Input: part model. Units: mm. Frame: model coordinates. A direction names the side the tool comes from. Coordinates: 2 decimals unless noted, no trailing zeros. Loops run counter-clockwise (first coordinate to the right, second up) from the corner with the lowest first, then second, coordinate; pieces in that order, holes last. Notation, with made-up numbers: (76.25, -5) - (125.25, -5) arc R13 ccw to (125.25, 4) - close; hole circle Ø5 at (88, 70.25). An arc over 180 degrees is marked (long way). Use one line per item in the form item = value.
from build123d import *

# Parameters (mm, degrees)
SCHIZZO1_W                    = 200
SCHIZZO1_H                    = 20
ESTRUSIONE_ESTRUSIONE1_DEPTH  = 25
SCHIZZO2_R                    = 2.25
TAGLIO_ESTRUSIONE1_DEPTH      = 141.400046302
SCHIZZO4_W                    = 2.020725942
SCHIZZO4_H                    = 10
SCHIZZO4_W_2                  = 2.598076211
SCHIZZO4_W_3                  = 3.175426481
TAGLIO_ESTRUSIONE2_DEPTH      = 1
SCHIZZO7_W                    = 15
SCHIZZO7_H                    = 5.5
TAGLIO_ESTRUSIONE3_DEPTH      = 141.400046302
SMUSSO1_SIZE                  = 1.5
SMUSSO1_SIZE2                 = 6
SCHIZZO8_W                    = 25
SCHIZZO8_H                    = 2.5
TAGLIO_ESTRUSIONE4_DEPTH      = 13
SCHIZZO9_W                    = 40
SCHIZZO9_H                    = 2.5
TAGLIO_ESTRUSIONE5_DEPTH      = 141.400046302
SCHIZZO10_W                   = 7
SCHIZZO10_H                   = 3
ESTRUSIONE_ESTRUSIONE5_DEPTH  = 4
SMUSSO2_SIZE                  = 4
SCHIZZO11_W                   = 2.5
SCHIZZO11_H                   = 8
TAGLIO_ESTRUSIONE6_DEPTH      = 141.400046302
SCHIZZO12_W                   = 6.5
SCHIZZO12_H                   = 6.5
TAGLIO_ESTRUSIONE7_DEPTH      = 4
SCHIZZO13_W                   = 9
SCHIZZO13_H                   = 10
ESTRUSIONE_ESTRUSIONE9_DEPTH  = 9
SCHIZZO14_W                   = 13
SCHIZZO14_H                   = 14
ESTRUSIONE_ESTRUSIONE10_DEPTH = 3.5
SMUSSO3_SIZE                  = 9
SMUSSO3_SIZE2                 = 4
SMUSSO4_SIZE                  = 4
SMUSSO4_SIZE2                 = 9
SCHIZZO16_R                   = 2.25
TAGLIO_ESTRUSIONE8_DEPTH      = 141.17038757
SCHIZZO17_R                   = 4
TAGLIO_ESTRUSIONE9_DEPTH      = 3


with BuildPart() as part:
    # Schizzo1 → Estrusione-Estrusione1 (new body)
    with BuildSketch(Plane.XY):
        with Locations((36.701035116, 4.318421053)):
            Rectangle(SCHIZZO1_W, SCHIZZO1_H)
    extrude(amount=ESTRUSIONE_ESTRUSIONE1_DEPTH)

    # Schizzo2 → Taglio-Estrusione1 (cut, through all)
    with BuildSketch(Plane(origin=(0, 14.318421053, 0), x_dir=(1, 0, 0), z_dir=(0, 1, 0))):
        with Locations(Location((-53.298964884, -15, 0), (0, 0, 270))):
            Circle(SCHIZZO2_R)
        Polygon((-23.80414637, -15.875), (-22.793783399, -15.875), (-22.288601913, -15), (-22.793783399, -14.125), (-23.80414637, -14.125), (-24.309327855, -15), align=None)
        Polygon((-14.999926779, -15), (-15.649445831, -13.875), (-16.948483937, -13.875), (-17.59800299, -15), (-16.948483937, -16.125), (-15.649445831, -16.125), align=None)
        Polygon((-8.505108264, -16.375), (-7.711251644, -15), (-8.505108264, -13.625), (-10.092821504, -13.625), (-10.886678125, -15), (-10.092821504, -16.375), align=None)
    extrude(amount=-TAGLIO_ESTRUSIONE1_DEPTH, mode=Mode.SUBTRACT)

    # Schizzo4 → Taglio-Estrusione2 (cut)
    with BuildSketch(Plane(origin=(0, 14.318421053, 0), x_dir=(1, 0, 0), z_dir=(0, 1, 0))):
        with Locations((-23.298964884, -20)):
            Rectangle(SCHIZZO4_W, SCHIZZO4_H)
        with Locations((-16.298964885, -20)):
            Rectangle(SCHIZZO4_W_2, SCHIZZO4_H)
        with Locations((-9.298964885, -20)):
            Rectangle(SCHIZZO4_W_3, SCHIZZO4_H)
    extrude(amount=-TAGLIO_ESTRUSIONE2_DEPTH, mode=Mode.SUBTRACT)

    # Schizzo7 → Taglio-Estrusione3 (cut, through all)
    with BuildSketch(Plane(origin=(0, 14.318421053, 0), x_dir=(1, 0, 0), z_dir=(0, 1, 0))):
        with Locations((14.788748356, -17.25)):
            Rectangle(SCHIZZO7_W, SCHIZZO7_H)
        with Locations((14.788748356, -7.75)):
            Rectangle(SCHIZZO7_W, SCHIZZO7_H)
    extrude(amount=-TAGLIO_ESTRUSIONE3_DEPTH, mode=Mode.SUBTRACT)

    # Smusso1
    smusso1_edges = [part.edges().sort_by_distance(p)[0] for p in [
        (14.788748356, 14.318421053, 14.5),
        (14.788748356, 14.318421053, 10.5),
    ]]
    smusso1_side = [part.faces().sort_by_distance(p)[0] for p in [
        (38.695689024, 14.318421053, 12.36530447),
    ]]
    chamfer(smusso1_edges, length=SMUSSO1_SIZE, length2=SMUSSO1_SIZE2, reference=smusso1_side[0])

    # Schizzo8 → Taglio-Estrusione4 (cut)
    with BuildSketch(Plane(origin=(0, 14.318421053, 0), x_dir=(1, 0, 0), z_dir=(0, 1, 0))):
        with Locations((49.788748356, -18.75)):
            Rectangle(SCHIZZO8_W, SCHIZZO8_H)
        with Locations((49.788748356, -11.25)):
            Rectangle(SCHIZZO8_W, SCHIZZO8_H)
    extrude(amount=-TAGLIO_ESTRUSIONE4_DEPTH, mode=Mode.SUBTRACT)

    # Schizzo9 → Taglio-Estrusione5 (cut, through all)
    with BuildSketch(Plane(origin=(0, 14.318421053, 0), x_dir=(1, 0, 0), z_dir=(0, 1, 0))):
        with Locations((116.701035116, -8.75)):
            Rectangle(SCHIZZO9_W, SCHIZZO9_H)
    extrude(amount=-TAGLIO_ESTRUSIONE5_DEPTH, mode=Mode.SUBTRACT)

    # Schizzo10 → Estrusione-Estrusione5 (add)
    with BuildSketch(Plane(origin=(0, 14.318421053, 0), x_dir=(1, 0, 0), z_dir=(0, 1, 0))):
        with Locations((133.201035116, -6)):
            Rectangle(SCHIZZO10_W, SCHIZZO10_H)
        with Locations((133.201035116, -11.5)):
            Rectangle(SCHIZZO10_W, SCHIZZO10_H)
    extrude(amount=ESTRUSIONE_ESTRUSIONE5_DEPTH)

    # Smusso2
    smusso2_edges = [part.edges().sort_by_distance(p)[0] for p in [
        (129.701035116, 18.318421053, 11.5),
        (129.701035116, 18.318421053, 6),
    ]]
    chamfer(smusso2_edges, length=SMUSSO2_SIZE - 0.0001)  # a hair under: the kernel refuses the full size

    # Schizzo11 → Taglio-Estrusione6 (cut, through all)
    with BuildSketch(Plane(origin=(0, 14.318421053, 0), x_dir=(1, 0, 0), z_dir=(0, 1, 0))):
        with Locations((99.951035116, -21)):
            Rectangle(SCHIZZO11_W, SCHIZZO11_H)
    extrude(amount=-TAGLIO_ESTRUSIONE6_DEPTH, mode=Mode.SUBTRACT)

    # Schizzo12 → Taglio-Estrusione7 (cut)
    with BuildSketch(Plane(origin=(0, 14.318421053, 0), x_dir=(1, 0, 0), z_dir=(0, 1, 0))):
        with Locations((99.951035116, -20.25)):
            Rectangle(SCHIZZO12_W, SCHIZZO12_H)
    extrude(amount=-TAGLIO_ESTRUSIONE7_DEPTH, mode=Mode.SUBTRACT)

    # Schizzo13 → Estrusione-Estrusione9 (add)
    with BuildSketch(Plane.XY.offset(25)):
        with Locations((29.788748356, -0.681578947)):
            Rectangle(SCHIZZO13_W, SCHIZZO13_H)
    extrude(amount=ESTRUSIONE_ESTRUSIONE9_DEPTH)

    # Schizzo14 → Estrusione-Estrusione10 (add)
    with BuildSketch(Plane.XY.offset(34)):
        with Locations((29.788748356, 1.318421053)):
            Rectangle(SCHIZZO14_W, SCHIZZO14_H)
    extrude(amount=ESTRUSIONE_ESTRUSIONE10_DEPTH)

    # Smusso3
    smusso3_edges = [part.edges().sort_by_distance(p)[0] for p in [
        (34.288748356, 4.318421053, 29.5),
    ]]
    smusso3_side = [part.faces().sort_by_distance(p)[0] for p in [
        (34.288748356, -0.681578947, 29.5),
    ]]
    chamfer(smusso3_edges, length=SMUSSO3_SIZE, length2=SMUSSO3_SIZE2, reference=smusso3_side[0])

    # Smusso4
    smusso4_edges = [part.edges().sort_by_distance(p)[0] for p in [
        (25.288748356, 4.318421053, 29.5),
    ]]
    smusso4_side = [part.faces().sort_by_distance(p)[0] for p in [
        (27.788748356, 4.318421053, 29.5),
    ]]
    chamfer(smusso4_edges, length=SMUSSO4_SIZE, length2=SMUSSO4_SIZE2, reference=smusso4_side[0])

    # Schizzo16 → Taglio-Estrusione8 (cut, through all)
    with BuildSketch(Plane.XY.offset(25)):
        with Locations((-37.648964884, 4.318421053)):
            Circle(SCHIZZO16_R)
        with Locations((79.451035116, 4.318421053)):
            Circle(SCHIZZO16_R)
    extrude(amount=-TAGLIO_ESTRUSIONE8_DEPTH, mode=Mode.SUBTRACT)

    # Schizzo17 → Taglio-Estrusione9 (cut)
    with BuildSketch(Plane.XY.offset(25)):
        with Locations((-37.648964884, 4.318421053)):
            Circle(SCHIZZO17_R)
        with Locations((79.451035116, 4.318421053)):
            Circle(SCHIZZO17_R)
    extrude(amount=-TAGLIO_ESTRUSIONE9_DEPTH, mode=Mode.SUBTRACT)


solid = part.part
Q1. Set-up query: faces 1 (the flat face through (23.289, 1, 36)), 2 (the flat face through (14.68, 11.28, 11.24)), 3 (the flat face through (116, 6, 7.5)), 4 (the flat face through (134, 16, 13)), 5 (the flat face through (15, 4, 5)). Return all of +Z, -Z, +X, -X, +Y, -Y with unobstructed straight access to the full face (end or side cutting, diameter ignored); none if empty.
Check values:
face_1 = +Z, -X, +Y, -Y
face_2 = +Y
face_3 = +X, +Y, -Y
face_4 = +Z, +X, -X, +Y
face_5 = +Y, -Y
Q2. Pull-direction query (Y, two-part tool) for faces 6 (the flat face through (35, -5.682, 14)), 7 (the flat face through (98.701, 2, 21)), 8 (the flat face through (35, 14.318, 12)), 9 (the cylindrical face through (-33.954, 2.786, 23.521)); classes: pulls with the +Y half, pulls with the -Y half, needs draft (parallel to the pull), parting line crosses it, or undercut.
Check values:
face_6 = pulls with the -Y half
face_7 = needs draft
face_8 = pulls with the +Y half
face_9 = undercut
Q3. Cut plane A-A, the plane z = 29.5. Return loops of the section in (x, y), then the cut area to 3 significant figures.
Check values:
outline = (25.29, -5.68) - (34.29, -5.68) - (34.29, -4.68) - (30.29, 4.32) - (29.29, 4.32) - (25.29, -4.68) - close
area = 54.0 mm²
Q4. Cut plane C-C, the plane y = -3. Give the number of separate pieces and of enclosed holes in the cut face, then the cut area to 3 significant figures.
Check values:
separate_pieces = 1
enclosed_holes = 6
area = 4,800 mm²
Q5. First-contact query: P1, Ø2, axis at x = 99.5, y = 14, coming from the -Z side; P2, Ø1.5, axis at x = 91.5, z = 7, coming from the +Y side; P3, Ø0.5, axis at y = -5, z = 29, coming from the -X side; P4, Ø8, axis at x = 103.5, y = 13, coming from the +Z side. Flat tips, straight axial feed; report the tip coordinate or a pass-through.
Check values:
P1 = 0
P2 = 14.32
P3 = 25.29
P4 = 25
Q6. Cut plane B-B, the plane x = -1.5. Return loops of the section in (y, z), then the cut area to 3 significant figures.
Check values:
outline = (-5.68, 0) - (14.32, 0) - (14.32, 25) - (-5.68, 25) - close
area = 500 mm²
Q7. Ray query, line 1 along X through (y, z) = (2, 15); line 2 along Z through (x, y) = (116, 9.25); line 3 along X through (y, z) = (5.25, 2.5). Return the intervals inside material, ascending. Write a range as [from, to].
Check values:
line_1 = [-63.3, -55.55], [-51.05, -24.31], [-22.29, -17.6], [-15, -10.89], [-7.71, 7.29], [22.29, 136.7]
line_2 = [0, 7.5], [10, 25]
line_3 = [-63.3, -39.7], [-35.6, 77.4], [81.5, 136.7]
